Input: dimensioned drawing with shaded views. Units: mm. Origin: part minimum x, y, z. A direction names the side the tool comes from. Round coordinates to 2 decimals unless told otherwise and drop trailing zeros. Order: outer loops, then holes, each group sorted by start corner. A loop starts at its lowest first (then second) coordinate and runs counter-clockwise, first axis right, second up. Notation, with made-up numbers: M 37.5,-29.5 L 72.5,-29.5 A5 cw 72.5,-24.5 Z; hole C -21.5,-29 d8. An arc over 180 degrees is marked long. One line per question, with ' | ' between items.
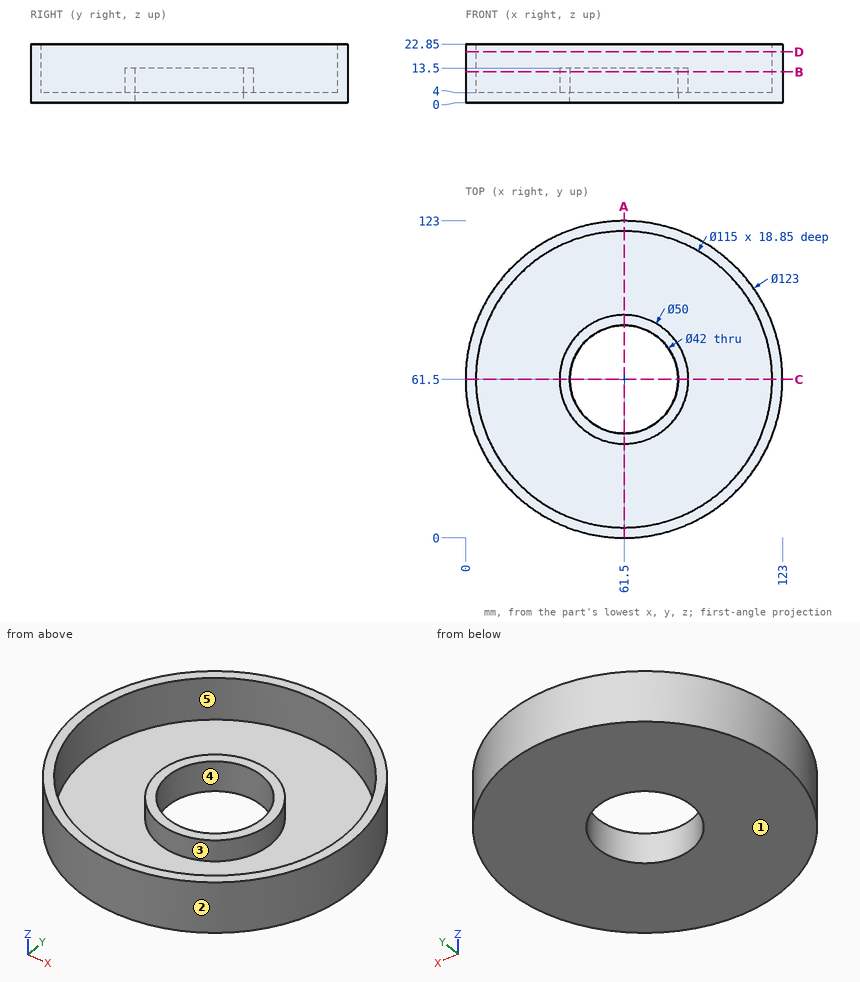
Item 1: Mould query, pull axis X, two halves, no side actions, for the marked faces 1, 2 and 3. Classes: +X half, -X half, draft (parallel to the pull), parting line (faces both ways), or undercut.
Report:
face 1: draft | face 2: parting line | face 3: undercut
Item 2: Section query D-D, the plane z = 19.75. Return loops of the section in (x, y).
Report:
outline: C 61.5,61.5 d123; hole C 61.5,61.5 d115
Item 3: First-contact query: pin 1 (1.5 mm diameter, centred on x = 46.5, y = 20.5, fed in from +Z); pin 2 (5 mm diameter, centred on y = 32, z = 19, fed in from -X); pin 3 (5 mm diameter, centred on y = 41.5, z = 20.5, fed in from -X). Flat tips, straight axial feed; report the tip coordinate or a pass-through.
Report:
pin 1: z = 4 | pin 2: x = 6.24 | pin 3: x = 2.54
Item 4: Section query A-A, the plane x = 61.5. Return loops of the section in (y, z).
Report:
outline: M 0,0 L 40.5,0 L 40.5,13.5 L 36.5,13.5 L 36.5,4 L 4,4 L 4,22.85 L 0,22.85 Z; M 82.5,0 L 123,0 L 123,22.85 L 119,22.85 L 119,4 L 86.5,4 L 86.5,13.5 L 82.5,13.5 Z
Item 5: Line query: line 1 along Y through (x, z) = (61.5, 9.75); line 2 along Y through (x, z) = (61.5, 18.5); line 3 along Z through (x, y) = (63, 8). Output: solid intervals per line, ascending. Write a range as from..to.
Report:
line 1: 0..4, 36.5..40.5, 82.5..86.5, 119..123 | line 2: 0..4, 119..123 | line 3: 0..4
Item 6: Section query B-B, the plane z = 12. Return loops of the section in (x, y).
Report:
outline: C 61.5,61.5 d123; C 61.5,61.5 d50; hole C 61.5,61.5 d115; hole C 61.5,61.5 d42
Item 7: Access query for the marked faces 4 and 5. Directions: +Z, -Z, +X, -X, +Y, -Y. A direction counts if a zero-diameter tool reaches every point of the face in a straight line with its end or side. Return the directions, or none.
Report:
face 4: +Z, -Z | face 5: +Z
